Work out the finished part from the listing and answer in its coordinate system (mm). A direction names the side the tool comes from. Round coordinates to 2 decimals unless told otherwise and drop trailing zeros. Write each loop counter-clockwise with the first axis right and the second up, starting at its lowest first coordinate (ties: lowest second). Pieces come first, ordered by that corner, then holes. Notation, with made-up numbers: M -8.75,77 L 41.25,77 A13 cw 41.25,89 Z; hole C 49.25,-39.75 d7. An arc over 180 degrees is marked long. One line per item, written item: value. Start each with the question number.
Q1. Find section C-C (y = 8.5). Write down the section's boundary in (x, z), and give its area (3 significant figures).
Q2. Find section D-D (z = -4.5). Write down the section's boundary in (x, y).
Q3. The mould has two halves that part along X. Classify faces 1 (the cylindrical face through (7.62, 6.59, -25.21)), 2 (the flat face through (-25, 5.5, 52)), 3 (the cylindrical face through (-52.75, 6.59, 54.78)): released by +X, released by -X, zero draft, split by the parting line, or undercut.
Q4. Find section A-A (y = 4.5). Write down the section's boundary in (x, z), and give its area (3 significant figures).
Q5. Given pin 1 Ø4.5 at (x, z) = (-49.18, -21.72) entering from -Y; pin 2 Ø12 at (x, z) = (-8, 10) entering from +Y, each flat-ended and moving along its own axis, determine where each tip first touches the part or whether it passes through.
Q6. Consider probe 1 along X at (y, z) = (12.75, 15); probe 2 along Z at (x, y) = (-2.5, 10.5); probe 3 along X at (y, z) = (11.5, -22). Determine where each line is inside the solid, lowest interval first.
Q7. Find section B-B (x = -19). Write down the section's boundary in (y, z), and give its area (3 significant figures).
Q8. A tool of negligible diameter and unlimited length cuts with its end or side. For faces 4 (the cylindrical face through (5.429, 1.528, -24.378)), 5 (the flat face through (-23, 0, 14)), 6 (the flat face through (-22, 8, -17.216)), from which of +Z, -Z, +X, -X, +Y, -Y can it reach the whole face along a straight path? Write none if from no direction.
Autodesk Fusion 360 part; units mm, degrees
sketch "Sketch1" plane through (0, 0, 0) normal (0, 1, 0) x (1, 0, 0)
  line L0 (-44.6765, -46.7839) -> (-0.4215, -46.7839)
  line L1 (-0.4215, -46.7839) -> (-0.4215, 17.2161)
  line L2 (-0.4215, 17.2161) -> (-44.6765, 17.2161)
  line L3 (-44.6765, 17.2161) -> (-44.6765, -46.7839)
  line L4 (-54.1765, -56.2839) -> (9.0449, -56.2839)
  line L5 (9.0449, -56.2839) -> (9.0449, 26.7161)
  line L6 (9.0449, 26.7161) -> (-54.1765, 26.7161)
  line L7 (-54.1765, 26.7161) -> (-54.1765, -56.2839)
  circle A0 centre (-49.1765, -51.2839) radius 1.7
  circle A1 centre (-49.1765, 21.7161) radius 1.7
  circle A2 centre (4.0449, 21.7161) radius 1.7
  circle A3 centre (4.0449, -51.2839) radius 1.7
  circle A4 centre (-49.1765, -51.2839) radius 3
  circle A5 centre (4.0449, -51.2839) radius 3
  circle A6 centre (4.0449, 21.7161) radius 3
  circle A7 centre (-49.1765, 21.7161) radius 3
  dimension "d1" = 64
  dimension "d2" = 83
  dimension "d3" = 9.5
  dimension "d4" = 9.5
  dimension "d5" = 3.4
  dimension "d6" = 5
  dimension "d7" = 5
  dimension "d8" = 3.4
  dimension "d9" = 63.2214
  dimension "d10" = 5
  dimension "d11" = 5
  dimension "d12" = 3.4
  dimension "d13" = 5
  dimension "d14" = 5
  dimension "d15" = 3.4
  dimension "d16" = 5
  dimension "d17" = 5
  dimension "d18" = 6
  dimension "d19" = 6
  dimension "d20" = 6
  dimension "d21" = 6
extrude "Extrude1" add sketch "Sketch1" along normal blind 9.9 from surface at 3.1 contours A4 | A5 | A6 | A7 makes body 1 at (-51.5679, 9.7, 49.4724) makes body 2 at (7.0412, 9.7, -21.5666) makes body 3 at (7.0412, 9.7, 51.4334) makes body 4 at (-46.1802, 9.7, -21.5666)
extrude "Extrude2" add sketch "Sketch1" along normal blind 13 contours L4 L5 L6 L7 bodies 1 2 3 4
extrude "Extrude3" add sketch "Sketch1" along normal blind 3 contours L0 L1 L2 L3 bodies 1
sketch "Sketch2" plane through (0, 13, 0) normal (0, 1, 0) x (-1, 0, 0)
  circle A0 centre (49.1765, 51.2839) radius 1.7
  circle A1 centre (49.1765, -21.7161) radius 1.7
  line L0 (44.6765, 46.7839) -> (44.6765, -17.2161)
  line L1 (44.6765, -17.2161) -> (0.4215, -17.2161)
  line L2 (0.4215, -17.2161) -> (0.4215, 46.7839)
  line L3 (0.4215, 46.7839) -> (44.6765, 46.7839)
  line L4 (54.1765, -26.7161) -> (54.1765, 56.2839)
  line L5 (54.1765, 56.2839) -> (-9.0449, 56.2839)
  line L6 (-9.0449, 56.2839) -> (-9.0449, -26.7161)
  line L7 (-9.0449, -26.7161) -> (54.1765, -26.7161)
  circle A2 centre (-4.0449, -21.7161) radius 1.7
  circle A3 centre (-4.0449, 51.2839) radius 1.7
  line L8 (15.3881, 56.2839) -> (33.8881, 56.2839)
  line L9 (33.8881, 56.2839) -> (33.8881, 46.7839)
  line L10 (33.8881, 46.7839) -> (15.3881, 46.7839)
  line L11 (15.3881, 46.7839) -> (15.3881, 56.2839)
  line L12 (-9.0449, 56.2839) -> (-9.0449, -26.7161)
  dimension "d29" = 18.5
  dimension "d30" = 24.433
extrude "Extrude4" cut sketch "Sketch2" against normal blind 7.5 contours L3 L5 L8 L9 L10 L11 bodies 1
fillet "Fillet1" radius 5 1 edges at (9.0449, 6.5, 56.2839) on bodies 1
fillet "Fillet2" radius 5 1 edges at (-54.1765, 6.5, 56.2839) on bodies 1
fillet "Fillet3" radius 5 1 edges at (-54.1765, 6.5, -26.7161) on bodies 1
fillet "Fillet4" radius 5 1 edges at (9.0449, 6.5, -26.7161) on bodies 1
The answers:
1. outline: M -54.18,-21.72 A5 ccw -49.18,-26.72 L 4.04,-26.72 A5 ccw 9.04,-21.72 L 9.04,51.28 A5 ccw 4.04,56.28 L -15.39,56.28 L -15.39,46.78 L -0.42,46.78 L -0.42,-17.22 L -44.68,-17.22 L -44.68,46.78 L -33.89,46.78 L -33.89,56.28 L -49.18,56.28 A5 ccw -54.18,51.28 Z; hole C -49.18,-21.72 d3.4; hole C -49.18,51.28 d3.4; hole C 4.04,-21.72 d3.4; hole C 4.04,51.28 d3.4
1. area: 2,180 mm2
2. outline: M -54.18,0 L 9.04,0 L 9.04,13 L -0.42,13 L -0.42,3 L -44.68,3 L -44.68,13 L -54.18,13 Z
3. face 1: released by +X
3. face 2: undercut
3. face 3: released by -X
4. outline: M -54.18,-21.72 A5 ccw -49.18,-26.72 L 4.04,-26.72 A5 ccw 9.04,-21.72 L 9.04,51.28 A5 ccw 4.04,56.28 L -49.18,56.28 A5 ccw -54.18,51.28 Z; hole C -49.18,-21.72 d3.4; hole C -49.18,51.28 d3.4; hole M -44.68,-17.22 L -0.42,-17.22 L -0.42,46.78 L -44.68,46.78 Z; hole C 4.04,-21.72 d3.4; hole C 4.04,51.28 d3.4
4. area: 2,360 mm2
5. pin 1: y = 3.1
5. pin 2: y = 3
6. probe 1: -54.18 to -44.68, -0.42 to 9.04
6. probe 2: -26.72 to -17.22, 46.78 to 56.28
6. probe 3: -54.17 to -50.85, -47.5 to 2.37, 5.72 to 9.04
7. outline: M 0,-26.72 L 13,-26.72 L 13,-17.22 L 3,-17.22 L 3,46.78 L 5.5,46.78 L 5.5,56.28 L 0,56.28 Z
7. area: 368 mm2
8. face 4: -Y
8. face 5: +Z, -Z, +X, -X, -Y
8. face 6: +Y
